```python
from build123d import *

# Parameters (mm, degrees)
F1_DEPTH  = 25
F1_TAPER  = 15
F2_R      = 10
F3_DEPTH  = 25
F8_DEPTH  = 25
F9_R      = 10
F10_DEPTH = 25
F11_R     = 10
F12_DEPTH = 25
F13_R     = 10
F5_DEPTH  = 25
F6_R      = 10
F7_DEPTH  = 25


with BuildPart() as f1:
    # F0 (on Top) → F1 (new body)
    with BuildSketch(Plane.XY):
        Polygon((-34.9069200456, 20.1535196849), (-34.9069200456, -20.1535196849), (0, -40.3070393698), (34.9069200456, -20.1535196849), (34.9069200456, 20.1535196849), (0, 40.3070393698), align=None)
    extrude(amount=F1_DEPTH, taper=F1_TAPER)

    # F2 (on face) → F3 (join)
    with BuildSketch(Plane(origin=(-16.2842998932, -28.2052347808, 8.7267300114), x_dir=(0.8756408079, -0.4613836487, 0.1427525977), z_dir=(-0.4829629131, -0.8365163037, 0.2588190451))):
        Circle(F2_R)
    extrude(amount=F3_DEPTH)

    # F4 (on face) → F8 (join)
    with BuildSketch(Plane(origin=(16.2842998932, -28.2052347808, 8.7267300114), x_dir=(0.8756408079, 0.4613836487, -0.1427525977), z_dir=(0.4829629131, -0.8365163037, 0.2588190451))):
        with BuildLine():
            ThreePointArc((5.5749073304, -8.3018316206), (8.8246550444, -4.7037711836), (10, 0))
            ThreePointArc((10, 0), (-5.9563004457, 8.0325889351), (-2.9044970001, -9.5689026109))
            Line((-2.9044970001, -9.5689026109), (5.5749073304, -8.3018316206))
        make_face()
    extrude(amount=F8_DEPTH)

    # F9 (on face) → F10 (join)
    with BuildSketch(Plane(origin=(32.5685997865, 0, 8.7267300114), x_dir=(0, 1, 0), z_dir=(0.9659258263, 0, 0.2588190451))):
        Circle(F9_R)
    extrude(amount=F10_DEPTH)

    # F11 (on face) → F12 (join)
    with BuildSketch(Plane(origin=(16.2842998932, 28.2052347808, 8.7267300114), x_dir=(-0.8756408079, 0.4613836487, 0.1427525977), z_dir=(0.4829629131, 0.8365163037, 0.2588190451))):
        Circle(F11_R)
    extrude(amount=F12_DEPTH)

    # F13 (on face) → F5 (join)
    with BuildSketch(Plane(origin=(-16.2842998932, 28.2052347808, 8.7267300114), x_dir=(-0.8756408079, -0.4613836487, -0.1427525977), z_dir=(-0.4829629131, 0.8365163037, 0.2588190451))):
        Circle(F13_R)
    extrude(amount=F5_DEPTH)

    # F6 (on face) → F7 (join)
    with BuildSketch(Plane(origin=(-32.5685997865, 0, 8.7267300114), x_dir=(0, -1, 0), z_dir=(-0.9659258263, 0, 0.2588190451))):
        Circle(F6_R)
    extrude(amount=F7_DEPTH)


solid = f1.part
```
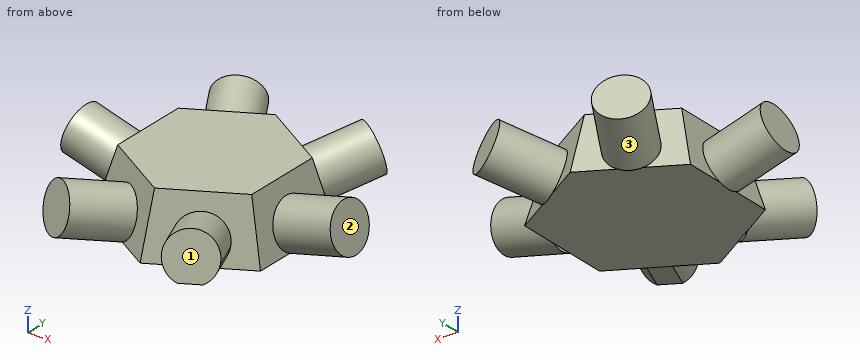
Could you check a few things on this model? Use its own coordinates, in mm. Face numbers are marked on the shaded views. Round coordinates to 2 decimals unless told otherwise and drop trailing zeros. Write each loop counter-clockwise with the first axis right and the second up, starting at its lowest first coordinate (ties: lowest second). Pieces come first, ordered by that corner, then holes. Notation, with made-up numbers: M 85,76.25 L 143,76.25 A18 cw 143,98.25 Z; hole C 65,46.5 d9. An arc over 180 degrees is marked long. Answer in a Markdown table with one row per item. Add a question column.
Q1. Imagine slicing it at C-C (x = -2). Please give me the cut outline in (y, z).
Q2. Imagine slicing it at B-B (z = 19.5). Give the number of separate pieces and of enclosed holes in the cut face, then the cut area to 3 significant figures.
Q3. Imagine slicing it at A-A (y = -6). Please give me the cut outline in (x, z).
Q4. If we mould it in two halves opening along Y, with no side actions, what happens to the marked faces 1, 2 and 3? For each: +Y half, -Y half, draft (parallel to the pull), parting line (faces both ways), or undercut.
Q5. Will these pins go through, and if not, where does the flat tip stop? pin 1 Ø4 at (y, z) = (-22.5, 9) entering from +X; pin 2 Ø12 at (x, z) = (7, 12.5) entering from -Y; pin 3 Ø1 at (y, z) = (-15.5, 8) entering from +X.
Q6. If I drill on line 1 (Y direction, x = 27.5, z = 14); line 2 (Z direction, x = -20.5, y = 16); line 3 (X direction, y = -50, z = 10.25), over which ranges is the centre line in solid material (lowest first)? Write a range as from..to.
Values:
| question | item | result |
|---|---|---|
| 1 | outline | M -39.15,0 L 39.15,0 L 31.42,25 L -31.42,25 Z |
| 2 | separate pieces | 7 |
| 2 | enclosed holes | 0 |
| 2 | area | 4,700 mm^2 |
| 3 | outline | M -58.79,7.47 L -34.64,1 L -34.91,0 L 34.91,0 L 34.64,1 L 58.79,7.47 L 54.65,22.92 L 30.5,16.45 L 28.21,25 L -28.21,25 L -30.5,16.45 L -54.65,22.92 Z |
| 4 | face 1 | -Y half |
| 4 | face 2 | draft |
| 4 | face 3 | undercut |
| 5 | pin 1 | x = 29.65 |
| 5 | pin 2 | y = -42.47 |
| 5 | pin 3 | x = 32.9 |
| 6 | line 1 | -49.98..-28.89, -20.1..20.1, 28.89..49.98 |
| 6 | line 2 | 0..25 |
| 6 | line 3 | -29.48..-18.12, 18.12..29.48 |
